```python
from build123d import *

# Parameters (mm, degrees)
ARA_D_ZLEM_R                    = 50
BASE_DEPTH                      = 5
Y_KSEKLIK_EKSTR_ZYON2_DEPTH     = 40
IZIM2_R                         = 2
BANANA_SLOTLAR_DEPTH            = 82.240384046
IZIM3_R                         = 2
IZIM3_R_2                       = 5.05
KES_EKSTR_ZYON1_DEPTH           = 5
IZIM3_2_R                       = 2
KES_EKSTR_ZYON2_DEPTH           = 82.240384046
IZIM5_R                         = 3.6
KES_EKSTR_ZYON3_DEPTH           = 79.89866919
IZIM6_R                         = 4.25
KES_EKSTR_ZYON4_DEPTH           = 7.5
PAH1_SIZE                       = 5
PAH1_SIZE2                      = 2
RADYUS1_R                       = 5
DAIRESEL_KAPLAMA1_COUNT         = 3
PAH1_OF_DAIRESEL_KAPLAMA1_SIZE2 = 2
PAH1_OF_DAIRESEL_KAPLAMA1_SIZE  = 5
RADYUS1_OF_DAIRESEL_KAPLAMA1_R  = 5


with BuildPart() as part:
    # ara d_zlem → base (new body)
    with BuildSketch(Plane(origin=(0, 0, 0), x_dir=(1, 0, 0), z_dir=(0, 1, 0))):
        with Locations(Location((0, 0, 0), (0, 0, 270))):
            Circle(ARA_D_ZLEM_R)
    extrude(amount=BASE_DEPTH)

    # izim1_3 → Y_kseklik-Ekstr_zyon2 (add)
    with BuildSketch(Plane(origin=(0, 0, 0), x_dir=(1, 0, 0), z_dir=(0, 1, 0))):
        with BuildLine():
            ThreePointArc((28.7, 40.942764929), (0, 50), (-28.7, 40.942764929))
            Line((-28.7, 40.942764929), (-28.7, -40.942764929))
            ThreePointArc((-28.7, -40.942764929), (0, -50), (28.7, -40.942764929))
            Line((28.7, -40.942764929), (28.7, 40.942764929))
        make_face()
    extrude(amount=Y_KSEKLIK_EKSTR_ZYON2_DEPTH)

    # izim2 → banana slotlar (cut, through all)
    with BuildSketch(Plane(origin=(0, 40, 0), x_dir=(1, 0, 0), z_dir=(0, 1, 0))):
        with Locations(Location((-11.3, -24.942764929, 0), (0, 0, 270))):
            Circle(IZIM2_R)
        with Locations(Location((-11.3, -36.942764929, 0), (0, 0, 90))):
            Circle(IZIM2_R)
    extrude(amount=-BANANA_SLOTLAR_DEPTH, mode=Mode.SUBTRACT)

    # izim3 → Kes-Ekstr_zyon1 (cut)
    with BuildSketch(Plane.XZ):
        with Locations(Location((-29.69848481, 29.69848481, 0), (0, 0, 270))):
            Circle(IZIM3_R)
        with Locations(Location((29.69848481, 29.69848481, 0), (0, 0, 270))):
            Circle(IZIM3_R)
        with Locations(Location((29.69848481, -29.69848481, 0), (0, 0, 270))):
            Circle(IZIM3_R)
        with Locations(Location((-29.69848481, -29.69848481, 0), (0, 0, 270))):
            Circle(IZIM3_R)
        with Locations(Location((0, 0, 0), (0, 0, 270))):
            Circle(IZIM3_R_2)
    extrude(amount=-KES_EKSTR_ZYON1_DEPTH, mode=Mode.SUBTRACT)

    # izim3_2 → Kes-Ekstr_zyon2 (cut, through all)
    with BuildSketch(Plane.XZ):
        with Locations(Location((-29.69848481, 29.69848481, 0), (0, 0, 270))):
            Circle(IZIM3_2_R)
        with Locations(Location((-29.69848481, -29.69848481, 0), (0, 0, 270))):
            Circle(IZIM3_2_R)
        with Locations(Location((29.69848481, -29.69848481, 0), (0, 0, 270))):
            Circle(IZIM3_2_R)
        with Locations(Location((29.69848481, 29.69848481, 0), (0, 0, 270))):
            Circle(IZIM3_2_R)
    extrude(amount=-KES_EKSTR_ZYON2_DEPTH, mode=Mode.SUBTRACT)

    # izim5 → Kes-Ekstr_zyon3 (cut, through all)
    with BuildSketch(Plane(origin=(0, 5, 0), x_dir=(1, 0, 0), z_dir=(0, 1, 0))):
        with Locations((29.69848481, -29.69848481)):
            Circle(IZIM5_R)
        with Locations((-29.69848481, -29.69848481)):
            Circle(IZIM5_R)
        with Locations((-29.69848481, 29.69848481)):
            Circle(IZIM5_R)
        with Locations((29.69848481, 29.69848481)):
            Circle(IZIM5_R)
    extrude(amount=KES_EKSTR_ZYON3_DEPTH, mode=Mode.SUBTRACT)

    # izim6 → Kes-Ekstr_zyon4 (cut)
    with BuildSketch(Plane(origin=(0, 40, 0), x_dir=(1, 0, 0), z_dir=(0, 1, 0))):
        with Locations(Location((0, -17.5, 0), (0, 0, 270))):
            Circle(IZIM6_R)
    kes_ekstr_zyon4 = extrude(amount=-KES_EKSTR_ZYON4_DEPTH, mode=Mode.SUBTRACT)

    # Pah1
    pah1_edges = [part.edges().sort_by_distance(p)[0] for p in [
        (0, 32.5, 13.25),
    ]]
    pah1_side = [part.faces().sort_by_distance(p)[0] for p in [
        (0, 36.25, 13.25),
    ]]
    chamfer(pah1_edges, length=PAH1_SIZE, length2=PAH1_SIZE2, reference=pah1_side[0])

    # Radyus1
    radyus1_edges = [part.edges().sort_by_distance(p)[0] for p in [
        (0, 37.5, 13.25),
    ]]
    fillet(radyus1_edges, radius=RADYUS1_R)

    # Dairesel Kaplama1: Kes-Ekstr_zyon4 ×3 about axis
    dairesel_kaplama1_axis = Axis((0, 0, 0), (0, 1, 0))
    for i in range(1, DAIRESEL_KAPLAMA1_COUNT):
        add(kes_ekstr_zyon4.rotate(dairesel_kaplama1_axis, i * 360 / DAIRESEL_KAPLAMA1_COUNT), mode=Mode.SUBTRACT)

    # Pah1 of Dairesel Kaplama1
    pah1_of_dairesel_kaplama1_edges = [part.edges().sort_by_distance(p)[0] for p in [
        (11.4748366, 32.5, -6.625),
        (-11.4748366, 32.5, -6.625),
    ]]
    chamfer(pah1_of_dairesel_kaplama1_edges, length=PAH1_OF_DAIRESEL_KAPLAMA1_SIZE, length2=PAH1_OF_DAIRESEL_KAPLAMA1_SIZE2)

    # Radyus1 of Dairesel Kaplama1
    radyus1_of_dairesel_kaplama1_edges = [part.edges().sort_by_distance(p)[0] for p in [
        (11.4748366, 37.5, -6.625),
        (-11.4748366, 37.5, -6.625),
    ]]
    fillet(radyus1_of_dairesel_kaplama1_edges, radius=RADYUS1_OF_DAIRESEL_KAPLAMA1_R)


solid = part.part
```
Can you work these out from the model? Positions are in its coordinate system, mm. A direction names the side the tool comes from. Coordinates: 2 decimals unless noted, no trailing zeros. Order: outer loops, then holes, each group sorted by start corner. A loop starts at its lowest first (then second) coordinate and runs counter-clockwise, first axis right, second up.
1. I'm going to push flat-ended pins straight in: pin 1 (4 mm diameter, centred on y = 29, z = -28, fed in from +X); pin 2 (8 mm diameter, centred on y = 8, z = -28, fed in from -X); pin 3 (6 mm diameter, centred on y = 14, z = -38, fed in from -X); pin 4 (6.5 mm diameter, centred on x = -29.7, z = -29.7, fed in from -Y). Where does each tip first touch, or does it pass through?
2. If we section it at A-A (y = 14): Please give me the cut outline in (x, z).
3. If we section it at B-B (z = 0): Please give me the cut outline in (x, y).
4. For faces 1 (the face through (26.1, 22.3, -29.8)), 2 (the face through (15, 32.5, -9)), 3 (the face through (-3.07, 2.46, 4.01)), which set-ups out of +Z, -Z, +X, -X, +Y, -Y let a thin tool reach every point of the face, with its end or its side?
5. I need wall thicknesses on line 1 (X direction, y = 39.4, z = 17.5); line 2 (Z direction, x = -12, y = 24); line 3 (Z direction, x = -27.5, y = 36). Which ranges of each line are inside material? Lowest first, please.
6. Thinking about a two-plate mould opening in Z: for faces 4 (the face through (0, 40, -1)), 5 (the face through (-28.35, 2.46, -28.22)), which applies, +Z half, -Z half, draft (parallel to the pull), parting line (faces both ways), or undercut?
7. If we section it at C-C (x = -43): Please give me the cut outline in (y, z), then the cut area to 3 significant figures.
8. If we section it at D-D (z = -21.5): Please give me the cut outline in (x, y), then the cut area to 3 significant figures.
Entries:
1. pin 1: stops at x = 28.7
1. pin 2: stops at x = -43.09
1. pin 3: stops at x = -28.7
1. pin 4: stops at y = 0
2. outline: (-28.7, -40.94) arc R50 ccw to (28.7, -40.94) - (28.7, -33.16) arc R3.6 cw to (28.7, -26.24) - (28.7, 26.24) arc R3.6 cw to (28.7, 33.16) - (28.7, 40.94) arc R50 ccw to (-28.7, 40.94) - (-28.7, 33.16) arc R3.6 cw to (-28.7, 26.24) - (-28.7, -26.24) arc R3.6 cw to (-28.7, -33.16) - close; hole circle Ø4 at (-11.3, 24.94); hole circle Ø4 at (-11.3, 36.94)
3. outline: (-50, 0) - (-5.05, 0) - (-5.05, 5) - (5.05, 5) - (5.05, 0) - (50, 0) - (50, 5) - (28.7, 5) - (28.7, 40) - (-28.7, 40) - (-28.7, 5) - (-50, 5) - close
4. face 1: +X, +Y
4. face 2: +Y
4. face 3: -Y
5. line 1: x = -28.7 to -4.25, 4.25 to 28.7
5. line 2: z = -48.54 to 23.07, 26.82 to 35.07, 38.82 to 48.54
5. line 3: z = -41.76 to -32.55, -26.85 to 26.85, 32.55 to 41.76
6. face 4: draft
6. face 5: undercut
7. outline: (0, -25.51) - (5, -25.51) - (5, 25.51) - (0, 25.51) - close
7. area: 255 mm2
8. outline: (-45.14, 0) - (45.14, 0) - (45.14, 5) - (28.7, 5) - (28.7, 40) - (-28.7, 40) - (-28.7, 5) - (-45.14, 5) - close
8. area: 2,460 mm2
